from build123d import *

# Parameters (mm, degrees)
BOSS_EXTRUDE1_DEPTH = 27
SKETCH2_R           = 8.75
BOSS_EXTRUDE2_DEPTH = 56
SKETCH3_R           = 8.75
BOSS_EXTRUDE3_DEPTH = 13
SKETCH4_R           = 5
BOSS_EXTRUDE4_DEPTH = 8
SKETCH6_R           = 2.5
CUT_EXTRUDE1_DEPTH  = 30
CUT_EXTRUDE2_REACH  = 107.929
SKETCH8_R           = 2.5
CUT_EXTRUDE3_DEPTH  = 106.929221653


with BuildPart() as part:
    # Sketch1 → Boss-Extrude1 (new body)
    with BuildSketch(Plane.XY):
        with BuildLine():
            ThreePointArc((-9, -4.358898944), (-7.071067812, -7.071067812), (-4.358898944, -9))
            Line((-4.358898944, -9), (4.358898944, -9))
            ThreePointArc((4.358898944, -9), (7.071067812, -7.071067812), (9, -4.358898944))
            Line((9, -4.358898944), (9, 4.358898944))
            ThreePointArc((9, 4.358898944), (7.071067812, 7.071067812), (4.358898944, 9))
            Line((4.358898944, 9), (-4.358898944, 9))
            ThreePointArc((-4.358898944, 9), (-7.071067812, 7.071067812), (-9, 4.358898944))
            Line((-9, 4.358898944), (-9, -4.358898944))
        make_face()
    extrude(amount=BOSS_EXTRUDE1_DEPTH)

    # Sketch2 → Boss-Extrude2 (add)
    with BuildSketch(Plane.XY.offset(27)):
        Circle(SKETCH2_R)
    extrude(amount=BOSS_EXTRUDE2_DEPTH)

    # Sketch3 → Boss-Extrude3 (add)
    # profile 1 of 2: a face of its own
    with BuildSketch(Plane.XY.offset(83)):
        with BuildLine():
            ThreePointArc((-9, -4.358898944), (-7.071067812, -7.071067812), (-4.358898944, -9))
            Line((-4.358898944, -9), (4.358898944, -9))
            ThreePointArc((4.358898944, -9), (7.071067812, -7.071067812), (9, -4.358898944))
            Line((9, -4.358898944), (9, 4.358898944))
            ThreePointArc((9, 4.358898944), (7.071067812, 7.071067812), (4.358898944, 9))
            Line((4.358898944, 9), (-4.358898944, 9))
            ThreePointArc((-4.358898944, 9), (-7.071067812, 7.071067812), (-9, 4.358898944))
            Line((-9, 4.358898944), (-9, -4.358898944))
        make_face()
        Circle(SKETCH3_R, mode=Mode.SUBTRACT)
    # profile 2 of 2: a face of its own
    with BuildSketch(Plane.XY.offset(83)):
        Circle(SKETCH3_R)
    extrude(amount=BOSS_EXTRUDE3_DEPTH)

    # Sketch4 → Boss-Extrude4 (add)
    with BuildSketch(Plane.XY.offset(96)):
        Circle(SKETCH4_R)
    extrude(amount=BOSS_EXTRUDE4_DEPTH)

    # Sketch6 → Cut-Extrude1 (cut)
    with BuildSketch(Plane.XY.offset(104)):
        Circle(SKETCH6_R)
    extrude(amount=-CUT_EXTRUDE1_DEPTH, mode=Mode.SUBTRACT)

    # Sketch7 → Cut-Extrude2 (cut, up to next)
    with BuildSketch(Plane(origin=(0, 9, 0), x_dir=(1, 0, 0), z_dir=(0, 1, 0)), mode=Mode.PRIVATE) as cut_extrude2_sk1:
        Polygon((0, 0), (-3.5, 0), (-3.5, -19), (3.5, -19), (3.5, 0), align=None)
    cut_extrude2_tool1 = extrude(cut_extrude2_sk1.sketch, amount=-CUT_EXTRUDE2_REACH, mode=Mode.PRIVATE) & part.part
    add(cut_extrude2_tool1.solids().sort_by_distance((0, 9, 9.5))[0], mode=Mode.SUBTRACT)

    # Sketch8 → Cut-Extrude3 (cut, through all)
    with BuildSketch(Plane.ZY.offset(9)):
        with Locations(Location((6, 0, 0), (0, 0, 270))):
            Circle(SKETCH8_R)
    extrude(amount=-CUT_EXTRUDE3_DEPTH, mode=Mode.SUBTRACT)


solid = part.part
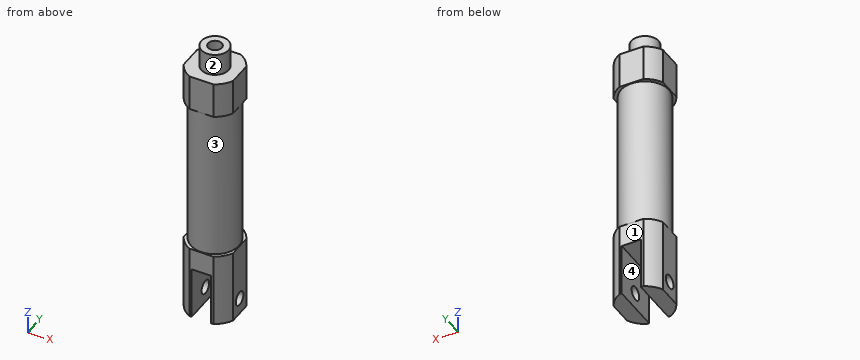
Check sheet for the modelled part. Datum: model origin and axes. Units: mm. Face numbers are marked on the shaded views. A direction names the side the tool comes from. Coordinates: 2 decimals unless noted, no trailing zeros. Loops run counter-clockwise (first coordinate to the right, second up) from the corner with the lowest first, then second, coordinate; pieces in that order, holes last. Notation, with made-up numbers: (32.25, -33.5) -> (50.25, -33.5) arc R28 ccw to (50.25, -3.5) -> close; hole circle Ø8 at (40, 77). An arc over 180 degrees is marked (long way). Answer in a Markdown table with one row per item.
1. Go/stop test with flat-tipped pins: pin 1 (1 mm diameter, centred on x = 0, z = 77.5, fed in from +Y); pin 2 (3.5 mm diameter, centred on x = 0.5, y = 1.5, fed in from -Z); pin 3 (6 mm diameter, centred on y = 7, z = 75, fed in from +X). Record where each tip stops, or that it passes through.
Check values:
| item | result |
|---|---|
| pin 1 | stops at y = 8.75 |
| pin 2 | stops at z = 19 |
| pin 3 | stops at x = 7.78 |
2. Material ranges on line 1 along Z through (x, y) = (7.55, 0); line 2 along Y through (x, z) = (0, 92.5); line 3 along X through (y, z) = (-2.5, 17.5), recorded low to high. Write a range as [from, to].
Check values:
| item | result |
|---|---|
| line 1 | z = [0, 3.5], [8.5, 96] |
| line 2 | y = [-9, -2.5], [2.5, 9] |
| line 3 | x = [-9, -3.5], [3.5, 9] |
3. Sectioned sample at B-B, the plane z = 6. Record the boundary of the cut face in (x, y).
Check values:
| item | result |
|---|---|
| outline | (-9, -4.36) arc R10 ccw to (-4.36, -9) -> (-3.5, -9) -> (-3.5, -2.5) -> (-9, -2.5) -> close; (-9, 2.5) -> (-3.5, 2.5) -> (-3.5, 9) -> (-4.36, 9) arc R10 ccw to (-9, 4.36) -> close; (3.5, -9) -> (4.36, -9) arc R10 ccw to (9, -4.36) -> (9, -2.5) -> (3.5, -2.5) -> close; (3.5, 2.5) -> (9, 2.5) -> (9, 4.36) arc R10 ccw to (4.36, 9) -> (3.5, 9) -> close |
4. Sectioned sample at D-D, the plane z = 90. Record the boundary of the cut face in (x, y), then the cut area to 3 significant figures.
Check values:
| item | result |
|---|---|
| outline | (-9, -4.36) arc R10 ccw to (-4.36, -9) -> (4.36, -9) arc R10 ccw to (9, -4.36) -> (9, 4.36) arc R10 ccw to (4.36, 9) -> (-4.36, 9) arc R10 ccw to (-9, 4.36) -> close; hole circle Ø5 at (0, 0) |
| area | 271 mm2 |
5. Access from +Z, -Z, +X, -X, +Y, -Y to the whole of each face (thin tool, end or side, straight path). Record for the marked faces 1 and 2.
Check values:
| item | result |
|---|---|
| face 1 | +Z, -Z, +X, -X, +Y |
| face 2 | +Z |
6. Release check for a two-part mould opening along Z. For the marked faces 3 and 4 record: released by +Z, released by -Z, zero draft, split by the parting line, or undercut.
Check values:
| item | result |
|---|---|
| face 3 | undercut |
| face 4 | zero draft |
7. Sectioned sample at C-C, the plane x = 0. Record the boundary of the cut face in (y, z).
Check values:
| item | result |
|---|---|
| outline | (-9, 19) -> (9, 19) -> (9, 27) -> (8.75, 27) -> (8.75, 83) -> (9, 83) -> (9, 96) -> (5, 96) -> (5, 104) -> (2.5, 104) -> (2.5, 74) -> (-2.5, 74) -> (-2.5, 104) -> (-5, 104) -> (-5, 96) -> (-9, 96) -> (-9, 83) -> (-8.75, 83) -> (-8.75, 27) -> (-9, 27) -> close |
8. Sectioned sample at A-A, the plane y = 0. Give the number of separate pieces and of enclosed holes in the cut face, then the cut area to 3 significant figures.
Check values:
| item | result |
|---|---|
| separate pieces | 3 |
| enclosed holes | 0 |
| area | 1,440 mm2 |
